from build123d import *

# Parameters (mm, degrees)
SKETCH1_R               = 65
SKETCH1_R_2             = 1.55
SKETCH1_R_3             = 16.5
BOSS_EXTRUDE1_DEPTH     = 10
SKETCH2_R               = 20
SKETCH2_R_2             = 16.1
BOSS_EXTRUDE2_DEPTH     = 70
BOSS_EXTRUDE3_START     = 35
SKETCH3_R               = 65
SKETCH3_R_2             = 45.25
BOSS_EXTRUDE3_DEPTH     = 35
SKETCH4_W               = 35
SKETCH4_H               = 35
BOSS_EXTRUDE4_DEPTH     = 35
SKETCH5_W               = 20.1
SKETCH5_H               = 20.1
CUT_EXTRUDE1_DEPTH      = 40
FILLET1_R               = 10
SKETCH6_R               = 2.05
CUT_EXTRUDE2_DEPTH      = 127
CUT_EXTRUDE3_DEPTH      = 1
CUT_EXTRUDE3_DEPTH_BACK = 16
SKETCH7_R               = 2.05


with BuildPart() as part:
    # Sketch1 → Boss-Extrude1 (new body)
    with BuildSketch(Plane.XY):
        Circle(SKETCH1_R)
        with Locations((-3.448790634, -40.478847481)):
            Circle(SKETCH1_R_2, mode=Mode.SUBTRACT)
        Circle(SKETCH1_R_3, mode=Mode.SUBTRACT)
        with Locations((-36.780105552, -17.252683439)):
            Circle(SKETCH1_R_2, mode=Mode.SUBTRACT)
        with Locations((-33.331314918, 23.226164042)):
            Circle(SKETCH1_R_2, mode=Mode.SUBTRACT)
        with Locations((3.448790634, 40.478847481)):
            Circle(SKETCH1_R_2, mode=Mode.SUBTRACT)
        with Locations((36.780105552, 17.252683439)):
            Circle(SKETCH1_R_2, mode=Mode.SUBTRACT)
        with Locations((33.331314918, -23.226164042)):
            Circle(SKETCH1_R_2, mode=Mode.SUBTRACT)
    extrude(amount=BOSS_EXTRUDE1_DEPTH)

    # Sketch2 → Boss-Extrude2 (add)
    with BuildSketch(Plane.XY.offset(10)):
        Circle(SKETCH2_R)
        Circle(SKETCH2_R_2, mode=Mode.SUBTRACT)
    extrude(amount=BOSS_EXTRUDE2_DEPTH)

    # Sketch3 → Boss-Extrude3 (add)
    with BuildSketch(Plane(origin=(0, 0, 0), x_dir=(-1, 0, 0), z_dir=(0, 0, -1)).offset(BOSS_EXTRUDE3_START)):
        Circle(SKETCH3_R)
        Circle(SKETCH3_R_2, mode=Mode.SUBTRACT)
    extrude(amount=-BOSS_EXTRUDE3_DEPTH)

    # Sketch4 → Boss-Extrude4 (add)
    with BuildSketch(Plane.XY.offset(10)):
        with Locations((-39.74569159, 0)):
            Rectangle(SKETCH4_W, SKETCH4_H)
        with Locations((40.25430841, 0)):
            Rectangle(SKETCH4_W, SKETCH4_H)
    extrude(amount=BOSS_EXTRUDE4_DEPTH)

    # Sketch5 → Cut-Extrude1 (cut)
    with BuildSketch(Plane(origin=(0, 17.5, 0), x_dir=(1, 0, 0), z_dir=(0, 1, 0))):
        with Locations((40.20430841, -27.45)):
            Rectangle(SKETCH5_W, SKETCH5_H)
        with Locations((-39.69569159, -27.45)):
            Rectangle(SKETCH5_W, SKETCH5_H)
    extrude(amount=-CUT_EXTRUDE1_DEPTH, mode=Mode.SUBTRACT)

    # Fillet1
    # the kernel refuses this fillet: 10 mm, written as the material it adds along each edge
    with BuildSketch(Plane(origin=(0, 0, 10), x_dir=(1, 0, 0), z_dir=(0, -1, 0))) as fillet1_piece_1:
        with BuildLine():
            CenterArc((20 + FILLET1_R, FILLET1_R), FILLET1_R, 180, 90)
            Line((20, FILLET1_R), (20, 0))
            Line((20, 0), (20 + FILLET1_R, 0))
        make_face()
    revolve(axis=Axis((0, 0, 10), (0, 0, 1)))

    # Sketch6 → Cut-Extrude2 (cut)
    with BuildSketch(Plane(origin=(57.75430841, 0, 0), x_dir=(0, 0, -1), z_dir=(1, 0, 0))):
        with Locations(Location((-27.5, 8.75, 0), (0, 0, 90))):
            Circle(SKETCH6_R)
        with Locations(Location((-27.5, -8.75, 0), (0, 0, 90))):
            Circle(SKETCH6_R)
    extrude(amount=-CUT_EXTRUDE2_DEPTH, mode=Mode.SUBTRACT)

    # Sketch7 → Cut-Extrude3 (cut, two sides: drawn at the far end of the back side and taken through both)
    with BuildSketch(Plane.XY.offset(45).offset(-CUT_EXTRUDE3_DEPTH_BACK)):
        with Locations((40.25430841, 8.5)):
            Circle(SKETCH7_R)
        with Locations((40.25430841, -9)):
            Circle(SKETCH7_R)
        with Locations((-40.25430841, -9)):
            Circle(SKETCH7_R)
        with Locations((-40.25430841, 8.5)):
            Circle(SKETCH7_R)
    extrude(amount=CUT_EXTRUDE3_DEPTH + CUT_EXTRUDE3_DEPTH_BACK, mode=Mode.SUBTRACT)


solid = part.part
Model file for the job. Use its own axes, mm. A direction names the side the tool comes from. Give positions to 0.01 mm unless a question says otherwise; leave off trailing zeros. Loops run counter-clockwise (first coordinate to the right, second up) from the corner with the lowest first, then second, coordinate; pieces in that order, holes last.
Item 1: Drop flat-ended pins along their axis: P1, Ø1.4, axis at x = 37.5, y = 16, coming from the -Z side; P2, Ø6.5, axis at x = -40.25, y = -9, coming from the +Z side; P3, Ø6.5, axis at y = -8.75, z = 27.5, coming from the -X side. Give the stop position or say it passes through.
Check values:
P1: stops at z = 0
P2: stops at z = 45
P3: stops at x = -57.25
Item 2: Slice it at C-C (y = 0). Give the number of separate pieces and of enclosed holes in the cut face, plus the area to 3 significant figures.
Check values:
separate pieces: 2
enclosed holes: 2
area: 4,570 mm2
Item 3: Drill centre lines: line 1 along Y through (x, z) = (0, 35); line 2 along Z through (x, y) = (-51.25, 8.75); line 3 along Y through (x, z) = (38.5, 16.5). Where is each one in solid material? Low to high.
Check values:
line 1: y = -20 to -16.1, 16.1 to 20
line 2: z = -35 to 25.45, 29.55 to 45
line 3: y = -17.5 to 17.5
Item 4: Slice it at A-A (x = 0). Write the cut outline in (y, z).
Check values:
outline: (-65, -35) - (-45.25, -35) - (-45.25, 0) - (-16.5, 0) - (-16.5, 10) - (-16.1, 10) - (-16.1, 80) - (-20, 80) - (-20, 20) arc R10 cw to (-30, 10) - (-65, 10) - close; (16.1, 10) - (16.5, 10) - (16.5, 0) - (45.25, 0) - (45.25, -35) - (65, -35) - (65, 10) - (30, 10) arc R10 cw to (20, 20) - (20, 80) - (16.1, 80) - close
Item 5: Slice it at B-B (z = 60). Write the cut outline in (x, y).
Check values:
outline: circle Ø40 at (0, 0); hole circle Ø32.2 at (0, 0)
Item 6: Which spindle directions (+Z, -Z, +X, -X, +Y, -Y) get a long thin tool onto all of the face, cutting with end or side? Do faces 4 (the face through (-40, 0, 45)), 5 (the face through (-49.746, 0, 28)), 6 (the face through (-43.16, 13.59, -17.74)), 7 (the face through (-40, -17.5, 16)), 8 (the face through (-38.3, 9.12, 41.2)). Say none if no direction does.
Check values:
face 4: +Z, -X, +Y, -Y
face 5: +Y, -Y
face 6: -Z
face 7: +Z, -X, -Y
face 8: +Z
Item 7: Mould opens along Y. For faces 1 (the face through (-14, 44, -35)), 2 (the face through (54.057, -10.261, 28.885)), 3 (the face through (-4.336, -19.524, 49.58)) say: +Y half, -Y half, draft (parallel to the pull), parting line (faces both ways), or undercut.
Check values:
face 1: draft
face 2: undercut
face 3: parting line
Item 8: Slice it at D-D (x = -27). Write the cut outline in (y, z), plus the area to 3 significant figures.
Check values:
outline: (-59.13, -35) - (-36.31, -35) - (-36.31, 0) - (36.31, 0) - (36.31, -35) - (59.13, -35) - (59.13, 10) - (17.5, 10) - (17.5, 45) - (-17.5, 45) - (-17.5, 10) - (-59.13, 10) - close; hole circle Ø4.1 at (-8.75, 27.5); hole circle Ø4.1 at (8.75, 27.5)
area: 3,980 mm2
